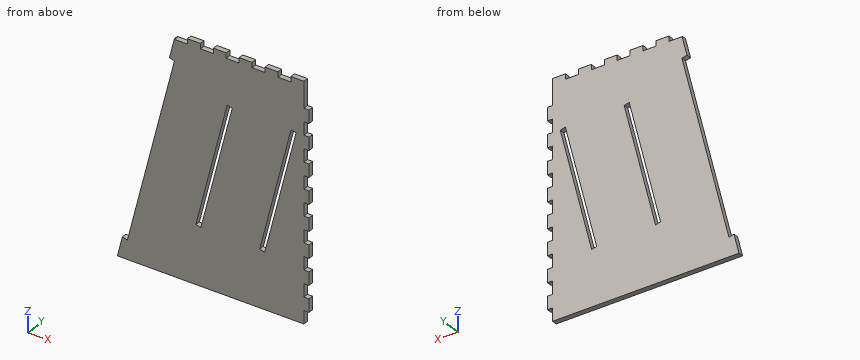
Autodesk Inventor part; units mm, degrees
ref_plane "YZ Plane" through (0, 0, 0) normal (1, 0, 0) x (0, 1, 0)
ref_plane "XZ Plane" through (0, 0, 0) normal (0, 1, 0) x (-1, 0, 0)
ref_plane "XY Plane" through (0, 0, 0) normal (0, 0, 1) x (1, 0, 0)
sketch "スケッチ1" plane through (0, 0, 0) normal (0, 1, 0) x (-1, 0, 0)
  line L0 (0, 0) -> (100, 0)
  line L1 (100, 0) -> (100, -180)
  line L2 (100, -180) -> (0, -180)
  line L3 (0, -180) -> (0, 0)
  line L4 (0, -170) -> (-4, -170)
  line L5 (-4, -170) -> (-4, -160)
  line L6 (-4, -160) -> (0, -160)
  line L7 (0, -160) -> (0, -170)
  line L8 (-4, -140) -> (0, -140)
  line L9 (-4, -150) -> (-4, -140)
  line L10 (0, -150) -> (-4, -150)
  line L11 (-4, -120) -> (0, -120)
  line L12 (-4, -130) -> (-4, -120)
  line L13 (0, -130) -> (-4, -130)
  line L14 (-4, -100) -> (0, -100)
  line L15 (-4, -110) -> (-4, -100)
  line L16 (0, -110) -> (-4, -110)
  line L17 (-4, -80) -> (0, -80)
  line L18 (-4, -90) -> (-4, -80)
  line L19 (0, -90) -> (-4, -90)
  line L20 (-4, -60) -> (0, -60)
  line L21 (-4, -70) -> (-4, -60)
  line L22 (0, -70) -> (-4, -70)
  line L23 (-4, -40) -> (0, -40)
  line L24 (-4, -50) -> (-4, -40)
  line L25 (0, -50) -> (-4, -50)
  line L26 (-4, -20) -> (0, -20)
  line L27 (-4, -30) -> (-4, -20)
  line L28 (0, -30) -> (-4, -30)
  line L29 (10, 0) -> (20, 0)
  line L30 (20, 0) -> (20, 4)
  line L31 (20, 4) -> (10, 4)
  line L32 (10, 4) -> (10, 0)
  line L33 (30, 4) -> (30, 0)
  line L34 (40, 4) -> (30, 4)
  line L35 (40, 0) -> (40, 4)
  line L36 (50, 4) -> (50, 0)
  line L37 (60, 4) -> (50, 4)
  line L38 (60, 0) -> (60, 4)
  line L39 (70, 4) -> (70, 0)
  line L40 (80, 4) -> (70, 4)
  line L41 (80, 0) -> (80, 4)
  line L42 (45, -180) -> (5, -20)
  line L43 (90.5, -180) -> (50.5, -20)
  line L44 (100, -20) -> (140, -180)
  line L45 (100, -180) -> (140, -180)
  line L46 (100, -3.5076) -> (144.2959, -180.6913)
  line L47 (140, -180) -> (144.1231, -180)
  line L48 (50.5, -20) -> (54.3806, -19.0299)
  line L49 (54.3806, -19.0299) -> (94.6231, -180)
  line L50 (5, -20) -> (1.1194, -20.9701)
  line L51 (1.1194, -20.9701) -> (40.8769, -180)
  line L52 (34.1043, -136.4171) -> (30.2237, -137.3872)
  line L53 (9.8507, -39.4029) -> (5.9701, -40.373)
  line L54 (55.3507, -39.4029) -> (59.2313, -38.4327)
  line L55 (79.6043, -136.4171) -> (83.4848, -135.447)
  line L56 (100, -20) -> (103.8806, -19.0299)
  line L57 (103.8806, -19.0299) -> (140.2609, -164.5512)
  line L58 (140.2609, -164.5512) -> (136.3803, -165.5214)
  line L59 (20, 0) -> (20, -4)
  line L60 (10, -4) -> (10, 0)
  line L61 (30, -4) -> (30, 0)
  line L62 (40, -4) -> (30, -4)
  line L63 (40, 0) -> (40, -4)
  line L64 (50, -4) -> (50, 0)
  line L65 (60, 0) -> (60, -4)
  line L66 (70, -4) -> (70, 0)
  line L67 (80, 0) -> (80, -4)
  line L68 (80, -4) -> (70, -4)
  line L69 (60, -4) -> (50, -4)
  line L70 (20, -4) -> (10, -4)
  line L71 (90, 0) -> (100, 0)
  line L72 (100, 0) -> (100, -4)
  line L73 (100, -4) -> (90, -4)
  line L74 (90, -4) -> (90, 0)
  point P0 (10, 2)
  point P1 (30, 2)
  point P2 (50, 2)
  point P3 (70, 2)
  point P4 (57.291, -38.9178)
  point P5 (0, -20)
  point P6 (0, -40)
  point P7 (0, -60)
  point P8 (0, -80)
  point P9 (0, -100)
  point P10 (0, -120)
  point P11 (0, -140)
  point P12 (0, -160)
  point P13 (50, -2)
  dimension "d0" = 100
  dimension "d1" = 180
  dimension "d2" = 4
  dimension "d3" = 10
  dimension "d4" = 10
  dimension "d7" = 20
  dimension "d12" = 10
  dimension "d13" = 4
  dimension "d14" = 10
  dimension "d17" = 20
  dimension "d22" = 45
  dimension "d23" = 5
  dimension "d24" = 20
  dimension "d26" = 45.5
  dimension "d27" = 45.5
  dimension "d28" = 20
  dimension "d29" = 49.5
  dimension "d30" = 49.5
  dimension "d32" = 4
  dimension "d33" = 4
  dimension "d34" = 4
  dimension "d35" = 20
  dimension "d36" = 100
  dimension "d37" = 20
  dimension "d38" = 100
  dimension "d39" = 150
  dimension "d42" = 10
  dimension "d43" = 4
  dimension "d44" = 10
extrude "押し出し1" add sketch "スケッチ1" along normal blind 4 contours L0 L60 L70 L59 L61 L62 L63 L64 L69 L65 L66 L68 L67 L74 L73 L1 L2 L49 L48 L43 L42 L50 L51 L3 | L3 L28 L27 L26 | L3 L25 L24 L23 | L3 L22 L21 L20 | L3 L19 L18 L17 | L3 L16 L15 L14 | L46 L56 L1 | L3 L13 L12 L11 | L44 L45 L1 | L46 L47 L44 L58 | L3 L10 L9 L8 | L2 L43 L55 L49 | L3 L4 L5 L6 | L2 L51 L52 L42 | L54 L43 L48 L49 | L53 L51 L50 L42
properties part number "ER_lipo_side_2" material "木材 (オーク)"
The listing builds one solid part. Answer for the finished solid, in the listing's coordinates (mm). Give positions to 0.01 mm unless a question says otherwise; leave off trailing zeros. Order: outer loops, then holes, each group sorted by start corner. A loop starts at its lowest first (then second) coordinate and runs counter-clockwise, first axis right, second up. Notation, with made-up numbers: (-9, 83) -> (44, 83) arc R16 cw to (44, 112) -> close; hole circle Ø1 at (17, -12). An arc over 180 degrees is marked (long way). One line per item, written item: value.
1) Find section A-A, the plane x = -27. Determine the outline of the cut face in (y, z).
Reported:
outline: (0, -180) -> (4, -180) -> (4, -124.49) -> (0, -124.49) -> close; (0, -108) -> (4, -108) -> (4, 0) -> (0, 0) -> close
2) Find section B-B, the plane z = -132. Determine the outline of the cut face in (x, y), plus the area to 3 significant figures.
Reported:
outline: (-128, 0) -> (-82.62, 0) -> (-82.62, 4) -> (-128, 4) -> close; (-78.5, 0) -> (-33, 0) -> (-33, 4) -> (-78.5, 4) -> close; (-28.88, 0) -> (0, 0) -> (0, 4) -> (-28.88, 4) -> close
area: 479 mm^2
3) Find the intervals of material crossed by line 1 (X direction, y = 0.9, z = -88); line 2 (X direction, y = 1.4, z = -124.5) (3 decimals); line 3 (Z direction, x = -91.5, y = 0.9), in increasing order.
Reported:
line 1: x = -117 to -71.62, -67.5 to -22, -17.88 to 4
line 2: x = -126.125 to -80.748, -76.625 to -31.125, -27.002 to 4
line 3: z = -180 to -4
4) Find section C-C, the plane z = -35. Determine the outline of the cut face in (x, y).
Reported:
outline: (-103.75, 0) -> (0, 0) -> (0, 4) -> (-103.75, 4) -> close
5) Flat-ended cylindrical pins translate along their axes: P1, Ø1.5, axis at x = -21, z = -39, coming from the -Y side; P2, Ø1.2, axis at x = -13.5, y = 2, coming from the +Z side; P3, Ø1.2, axis at x = 1.5, y = 1.5, coming from the -Z side; P4, Ø1.2, axis at x = 1.5, y = 1.5, coming from the +Z side. Find the tip coordinate at first contact, or state that the pin passes through.
Reported:
P1: stops at y = 0
P2: stops at z = -4
P3: stops at z = -170
P4: stops at z = -20
6) Find section D-D, the plane z = -64. Determine the outline of the cut face in (x, y).
Reported:
outline: (-111, 0) -> (-65.62, 0) -> (-65.62, 4) -> (-111, 4) -> close; (-61.5, 0) -> (-16, 0) -> (-16, 4) -> (-61.5, 4) -> close; (-11.88, 0) -> (4, 0) -> (4, 4) -> (-11.88, 4) -> close
